Autodesk Inventor part; units mm, degrees
ref_plane "YZ Plane" through (0, 0, 0) normal (1, 0, 0) x (0, 1, 0)
ref_plane "XZ Plane" through (0, 0, 0) normal (0, 1, 0) x (-1, 0, 0)
ref_plane "XY Plane" through (0, 0, 0) normal (0, 0, 1) x (1, 0, 0)
sketch "Sketch1" plane through (0, 0, 0) normal (0, 0, 1) x (1, 0, 0)
  circle A0 centre (0, 0) radius 12.5
  dimension "d0" = 25
extrude "Extrusion1" add sketch "Sketch1" along normal blind 3.75
sketch "Sketch2" plane through (0, 0, 3.75) normal (0, 0, 1) x (1, 0, 0)
  circle A0 centre (0, 0) radius 12.5
  circle A1 centre (0, 0) radius 6.35
  dimension "d3" = 12.7
extrude "Extrusion2" add sketch "Sketch2" along normal blind 14 contours A1
sketch "Sketch3" plane through (0, 0, 17.75) normal (0, 0, 1) x (1, 0, 0)
  circle A0 centre (0, 0) radius 6.35
hole "Hole1" at (0, 0, 17.75) direction (0, 0, -1) diameter 8 end through all
sketch "Sketch4" plane through (0, 0, 3.75) normal (0, 0, 1) x (1, 0, 0)
  circle A0 centre (0, 0) radius 12.5
  line L0 (-7.9971, -4.6239) -> (-0.0058, 9.2376) construction
  line L1 (-0.0058, 9.2376) -> (8.0029, -4.6137) construction
  line L2 (8.0029, -4.6137) -> (-7.9971, -4.6239) construction
  circle A1 centre (0, 0) radius 9.2376 construction
  dimension "d13" = 16
hole "Hole2" at (-7.9971, -4.6239, 3.75) at (-0.0058, 9.2376, 3.75) at (8.0029, -4.6137, 3.75) direction (0, 0, -1) diameter 2.459 end through all
fillet "Fillet1" radius 0.5 2 edges at (-12.5, 0, 3.75) (-6.35, 0, 17.75)
properties part number "lead carriage"
Can you work these out from the model? Positions are in its coordinate system, mm. A direction names the side the tool comes from. Coordinates: 2 decimals unless noted, no trailing zeros. Loops run counter-clockwise (first coordinate to the right, second up) from the corner with the lowest first, then second, coordinate; pieces in that order, holes last. Notation, with made-up numbers: M -32,-5 L -17,-5 A26 cw -17,28 Z; hole C -4,6 d6. An arc over 180 degrees is marked long. Answer as CSV lines item,"result". Start each with the question number.
1. Suppose I cut it at A-A, the plane y = 0. List the corners of the cut face in (x, z) for me.
2. Suppose I cut it at B-B, the plane z = 14.5. List the corners of the cut face in (x, y) for me, plus the area to 3 significant figures.
3. Thinking about a two-plate mould opening in X: for faces 1 (the face through (3, -4, 17.75)), 2 (the face through (-1.38, 6.2, 10.41)), 3 (the face through (7.17, -3.71, 1.85)), which applies, +X half, -X half, draft (parallel to the pull), parting line (faces both ways), or undercut?
4. For faces 4 (the face through (5, -5, 3.75)), 5 (the face through (3.905, 0.867, 8.751)), which set-ups out of +Z, -Z, +X, -X, +Y, -Y let a thin tool reach every point of the face, with its end or its side?
5. If I drill on probe 1 along X at (y, z) = (1.25, 11); probe 2 along X at (y, z) = (3.25, 9.75); probe 3 along Z at (x, y) = (-4.5, 6), over which ranges is the centre line in solid material (lowest first)? Write a range as [from, to].
6. For pin 1 Ø4 at (x, y) = (-0.01, 9.24) entering from +Z; pin 2 Ø8 at (x, z) = (-5, 3.5) entering from -Y; pin 3 Ø3 at (y, z) = (6, 10) entering from -X, each with a flat end and sliding along its axis, tell me the tip position at first contact or that it passes through.
Output:
1,outline,"M -12.5,0 L -4,0 L -4,17.75 L -5.85,17.75 A0.5 ccw -6.35,17.25 L -6.35,3.75 L -12,3.75 A0.5 ccw -12.5,3.25 Z; M 4,0 L 12.5,0 L 12.5,3.25 A0.5 ccw 12,3.75 L 6.35,3.75 L 6.35,17.25 A0.5 ccw 5.85,17.75 L 4,17.75 Z"
2,outline,"C 0,0 d12.7; hole C 0,0 d8"
2,area,"76.4 mm^2"
3,face 1,"draft"
3,face 2,"parting line"
3,face 3,"undercut"
4,face 4,"+Z"
4,face 5,"+Z, -Z"
5,probe 1,"x = [-6.23, -3.8], [3.8, 6.23]"
5,probe 2,"x = [-5.46, -2.33], [2.33, 5.46]"
5,probe 3,"z = [0, 3.75]"
6,pin 1,"stops at z = 3.75"
6,pin 2,"stops at y = -12.46"
6,pin 3,"stops at x = -4.48"
